Design review of the part built by this model. Coordinates are the model's own, in mm. Face numbers are marked on the shaded views. A direction names the side the tool comes from. Coordinates: 2 decimals unless noted, no trailing zeros. Loops run counter-clockwise (first coordinate to the right, second up) from the corner with the lowest first, then second, coordinate; pieces in that order, holes last. Notation, with made-up numbers: (-36.75, 71) -> (-29.75, 71) arc R22 cw to (-29.75, 86) -> close; hole circle Ø9 at (15, 84.5). An arc over 180 degrees is marked (long way). Answer as a JSON object with one key per item and string values.
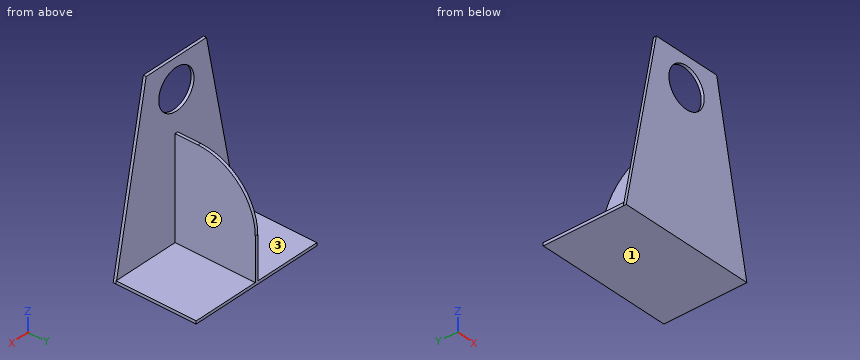
```python
from build123d import *

# Parameters (mm, degrees)
F3_DEPTH = 6.35
F4_D     = 89.1794
F5_W     = 304.8
F5_H     = 177.8
F6_DEPTH = 6.35
F7_W     = 3.175
F7_H     = 221.1080746889
F8_DEPTH = 177.8
F9_R     = 127


# Not quite as in the source:
# - a variable given as a bare number and used for a length is read in inches; the dataset says mm whatever the document's units were


with BuildPart() as f3:
    # F1 (on Front) → F3 (new body)
    with BuildSketch(Plane.XZ):
        Polygon((129.7632297397, 381), (-22.6367702603, 381), (-98.8367702603, 0), (205.9632297397, 0), align=None)
    extrude(amount=F3_DEPTH)

    # F4 (through all)
    with Locations(Plane(origin=(0, 0, 0), x_dir=(1, 0, 0), z_dir=(0, 1, 0))):
        with Locations((53.5632297397, -315.9252)):
            Hole(F4_D / 2)

    # F5 (on Top) → F6 (join)
    with BuildSketch(Plane.XY):
        with Locations((53.5632297397, 88.9)):
            Rectangle(F5_W, F5_H)
    extrude(amount=F6_DEPTH)

    # F7 (on face) → F8 (join)
    with BuildSketch(Plane(origin=(0, 0, 0), x_dir=(-1, 0, 0), z_dir=(0, 1, 0))):
        with Locations((-55.1507297397, 116.9040373445)):
            Rectangle(F7_W, F7_H)
        with Locations((-51.9757297397, 116.9040373445)):
            Rectangle(F7_W, F7_H)
    extrude(amount=F8_DEPTH)

    # F9
    f9_edges = [f3.edges().sort_by_distance(p)[0] for p in [
        (53.56323, 177.8, 227.458075),
    ]]
    fillet(f9_edges, radius=F9_R)


solid = f3.part
```
1) Clearance check with flat-ended pins moving along their axes: pin 1 Ø2 at (y, z) = (145, 156.5) entering from -X; pin 2 Ø3 at (x, y) = (54.5, 21.5) entering from +Z; pin 3 Ø1 at (x, y) = (125.5, 29.5) entering from +Z. State where each tip first meets the part, or that it passes through.
Completed:
{"pin 1": "x = 50.39", "pin 2": "z = 227.46", "pin 3": "z = 6.35"}
2) Wall thickness on probe 1 along X at (y, z) = (156, 33); probe 2 along Y at (x, z) = (58, 47); probe 3 along Z at (x, y) = (49, 146.5): over which ranges is each line inside the solid? List them lowest first.
Completed:
{"probe 1": "50.39 to 56.74", "probe 2": "-6.35 to 0", "probe 3": "0 to 6.35"}
3) Add section A-A, the plane y = 11.5. Give the boundary of the cut face in (x, z).
Completed:
{"outline": "(-98.84, 0) -> (205.96, 0) -> (205.96, 6.35) -> (56.74, 6.35) -> (56.74, 227.46) -> (50.39, 227.46) -> (50.39, 6.35) -> (-98.84, 6.35) -> close"}
4) Add section B-B, the plane x = -16. Give the boundary of the cut face in (y, z), and give its area (3 significant figures).
Completed:
{"outline": "(-6.35, 0) -> (177.8, 0) -> (177.8, 6.35) -> (0, 6.35) -> (0, 381) -> (-6.35, 381) -> close", "area": "3,550 mm²"}
5) For the marked faces 1, 2 and 3, list the 3-axis set-ups (+Z, -Z, +X, -X, +Y, -Y) from which the entire face can be reached by the end or side of a thin tool; tool diameter is ignored.
Completed:
{"face 1": "-Z, +X, -X, +Y, -Y", "face 2": "+Z, +X, +Y", "face 3": "+Z, -X, +Y"}
6) Add section D-D, the plane z = 168. Give the boundary of the cut face in (x, y), and give its area (3 significant figures).
Completed:
{"outline": "(-65.24, -6.35) -> (172.36, -6.35) -> (172.36, 0) -> (56.74, 0) -> (56.74, 158.35) -> (50.39, 158.35) -> (50.39, 0) -> (-65.24, 0) -> close", "area": "2,510 mm²"}
7) Add section C-C, the plane z = 278.5. Give the boundary of the cut face in (x, y).
Completed:
{"outline": "(-43.14, -6.35) -> (29.32, -6.35) -> (29.32, 0) -> (-43.14, 0) -> close; (77.8, -6.35) -> (150.26, -6.35) -> (150.26, 0) -> (77.8, 0) -> close"}
